from build123d import *

# Parameters (mm, degrees)
SKETCH2_R               = 5.156250121
BOSS_EXTRUDE1_DEPTH     = 10
SKETCH3_R               = 3.85
BOSS_EXTRUDE2_DEPTH     = 6.5
CUT_EXTRUDE1_DEPTH      = 19.039507494
CUT_EXTRUDE1_DEPTH_BACK = 19.039507494
SKETCH5_R               = 0.8


with BuildPart() as part:
    # Sketch2 → Boss-Extrude1 (new body)
    with BuildSketch(Plane.XY):
        Circle(SKETCH2_R)
    extrude(amount=-BOSS_EXTRUDE1_DEPTH)

    # Sketch3 → Boss-Extrude2 (add)
    with BuildSketch(Plane(origin=(0, 0, -10), x_dir=(-1, 0, 0), z_dir=(0, 0, -1))):
        with Locations(Location((0, 0, 0), (0, 0, 180))):
            Circle(SKETCH3_R)
    extrude(amount=BOSS_EXTRUDE2_DEPTH)

    # Sketch5 → Cut-Extrude1 (cut, two sides: drawn at the far end of the back side and taken through both)
    with BuildSketch(Plane.XY.offset(-CUT_EXTRUDE1_DEPTH_BACK)):
        Circle(SKETCH5_R)
    extrude(amount=CUT_EXTRUDE1_DEPTH + CUT_EXTRUDE1_DEPTH_BACK, mode=Mode.SUBTRACT)


solid = part.part
Verification items for the finished model (mm, model axes). A direction names the side the tool comes from. Round coordinates to 2 decimals unless told otherwise and drop trailing zeros. Loops run counter-clockwise (first coordinate to the right, second up) from the corner with the lowest first, then second, coordinate; pieces in that order, holes last. Notation, with made-up numbers: (27.25, 65.5) - (53.25, 65.5) arc R22 ccw to (53.25, 95.5) - close; hole circle Ø4 at (23, -35.5). An arc over 180 degrees is marked (long way). Answer in a Markdown table with one row per item. Add a question column.
Q1. Release check for a two-part mould opening along X. For faces 1 (the face through (-0.63, -0.49, -8.37)), 2 (the face through (-1.118, -5.034, -4.93)), 3 (the face through (1, 0, 0)) record: pulls with the +X half, pulls with the -X half, needs draft (parallel to the pull), parting line crosses it, or undercut.
Q2. Section check C-C on z = -8.75. Enter the section's corners in (x, y), plus the area to 3 significant figures.
Q3. Material ranges on line 1 (Y direction, x = 0, z = -4); line 2 (Y direction, x = 0, z = -10.5); line 3 (Z direction, x = 1.25, y = 4), recorded low to high.
Q4. Section check A-A on y = 0. Enter the section's corners in (x, z).
Q5. Section check D-D on x = 2. Enter the section's corners in (y, z).
Q6. Gauge pin test, flat ends, axial feed: pin 1 (5 mm diameter, centred on x = 3.5, z = -12, fed in from -Y); pin 2 (5 mm diameter, centred on x = -2, z = -7.5, fed in from -Y); pin 3 (1.5 mm diameter, centred on y = 3, z = -12, fed in from -X); pin 4 (2 mm diameter, centred on y = -4, z = -14, fed in from +X). Record the tip position at first contact, or that the pin passes through.
Q7. Tool access check on faces 4 (the face through (4, -1, -10)), 5 (the face through (0, 1, -16.5)). Record the directions out of +Z, -Z, +X, -X, +Y, -Y that give a thin tool (end or side, any length) a straight path to the whole face; none if there is none.
Found:
| question | item | result |
|---|---|---|
| 1 | face 1 | undercut |
| 1 | face 2 | parting line crosses it |
| 1 | face 3 | needs draft |
| 2 | outline | circle Ø10.31 at (0, 0); hole circle Ø1.6 at (0, 0) |
| 2 | area | 81.5 mm² |
| 3 | line 1 | y = -5.16 to -0.8, 0.8 to 5.16 |
| 3 | line 2 | y = -3.85 to -0.8, 0.8 to 3.85 |
| 3 | line 3 | z = -10 to 0 |
| 4 | outline | (-5.16, -10) - (-3.85, -10) - (-3.85, -16.5) - (-0.8, -16.5) - (-0.8, 0) - (-5.16, 0) - close; (0.8, -16.5) - (3.85, -16.5) - (3.85, -10) - (5.16, -10) - (5.16, 0) - (0.8, 0) - close |
| 5 | outline | (-4.75, -10) - (-3.29, -10) - (-3.29, -16.5) - (3.29, -16.5) - (3.29, -10) - (4.75, -10) - (4.75, 0) - (-4.75, 0) - close |
| 6 | pin 1 | stops at y = -4.75 |
| 6 | pin 2 | stops at y = -5.16 |
| 6 | pin 3 | stops at x = -3.12 |
| 6 | pin 4 | stops at x = 2.41 |
| 7 | face 4 | -Z |
| 7 | face 5 | -Z, +X, -X, +Y, -Y |
